```python
from build123d import *

# Parameters (mm, degrees)
SKETCH1_R           = 20
BOSS_EXTRUDE1_DEPTH = 30
SKETCH2_R           = 20
BOSS_EXTRUDE2_DEPTH = 5
SKETCH3_R           = 5.5
BOSS_EXTRUDE3_DEPTH = 5
FILLET1_R           = 10


with BuildPart() as part:
    # Sketch1 → Boss-Extrude1 (new body)
    with BuildSketch(Plane(origin=(0, 0, 0), x_dir=(1, 0, 0), z_dir=(0, 1, 0))):
        Circle(SKETCH1_R)
        with BuildLine():
            Line((-4.4, 17.6), (4.4, 17.6))
            Line((4.4, 17.6), (4.4, 12.073214154))
            ThreePointArc((4.4, 12.073214154), (0, -12.85), (-4.4, 12.073214154))
            Line((-4.4, 12.073214154), (-4.4, 17.6))
        make_face(mode=Mode.SUBTRACT)
    extrude(amount=BOSS_EXTRUDE1_DEPTH)

    # Sketch2 → Boss-Extrude2 (add)
    with BuildSketch(Plane(origin=(0, 30, 0), x_dir=(1, 0, 0), z_dir=(0, 1, 0))):
        Circle(SKETCH2_R)
    extrude(amount=BOSS_EXTRUDE2_DEPTH)

    # Sketch3 → Boss-Extrude3 (add)
    with BuildSketch(Plane(origin=(0, 35, 0), x_dir=(1, 0, 0), z_dir=(0, 1, 0))):
        Circle(SKETCH3_R)
        with BuildLine():
            Line((-2.71339271, 1.6), (2.71339271, 1.6))
            ThreePointArc((2.71339271, 1.6), (0, -3.15), (-2.71339271, 1.6))
        make_face(mode=Mode.SUBTRACT)
    extrude(amount=BOSS_EXTRUDE3_DEPTH)

    # Fillet1
    fillet1_edges = [part.edges().sort_by_distance(p)[0] for p in [
        (-20, 35, 0),
    ]]
    fillet(fillet1_edges, radius=FILLET1_R)


solid = part.part
```
Input: part model. Units: mm. Frame: model coordinates. A direction names the side the tool comes from. Give positions to 0.01 mm unless a question says otherwise; leave off trailing zeros. Write each loop counter-clockwise with the first axis right and the second up, starting at its lowest first coordinate (ties: lowest second). Pieces come first, ordered by that corner, then holes. Notation, with made-up numbers: (84, 70.5) - (98, 70.5) arc R28 ccw to (98, 106.5) - close; hole circle Ø3 at (31, 25). An arc over 180 degrees is marked (long way). Write item = value, one per line. Start each with the question number.
1. Ray query, L1, parallel to X at y = 14, z = 0; L2, parallel to Z at x = 0, y = 11.75; L3, parallel to Z at x = 0, y = 38.25. Return the intervals inside material, ascending.
2. First-contact query: pin 1 Ø15.5 at (x, z) = (0, 0) entering from -Y; pin 2 Ø5 at (x, z) = (10, -9.5) entering from +Y; pin 3 Ø4.5 at (x, y) = (1.5, 20.5) entering from +Z. Flat tips, straight axial feed; report the tip coordinate or a pass-through.
3. Access query for faces 5 (the cylindrical face through (0.09, 37.47, 3.15)), 6 (the flat face through (0, 15, -17.6)), 7 (the flat face through (-0.3, 0, 13.1)). Directions: +Z, -Z, +X, -X, +Y, -Y. A direction counts if a zero-diameter tool reaches every point of the face in a straight line with its end or side. Return the directions, or none.
4. Section query A-A, the plane y = 11. Output: boundary loops of the cut face in (x, z).
5. Mould query, pull axis X, two halves, no side actions, for faces 1 (the cylindrical face through (-4.336, 12.325, 19.524)), 2 (the cylindrical face through (0.5, 14.79, 12.84)), 3 (the flat face through (0, 30, -3)), 4 (the flat face through (0, 40, -3)). Classes: released by +X, released by -X, zero draft, split by the parting line, or undercut.
Check sheet entries:
q1.L1 = -20 to -12.85, 12.85 to 20
q1.L2 = -20 to -17.6, 12.85 to 20
q1.L3 = -5.5 to -1.6, 3.15 to 5.5
q2.pin_1 = 30
q2.pin_2 = 34.92
q2.pin_3 = 20
q3.face_5 = +Y
q3.face_6 = -Y
q3.face_7 = +Z, -Z, +X, -X, -Y
q4.outline = circle Ø40 at (0, 0); hole (-4.4, -17.6) - (4.4, -17.6) - (4.4, -12.07) arc R12.85 ccw (long way) to (-4.4, -12.07) - close
q5.face_1 = split by the parting line
q5.face_2 = undercut
q5.face_3 = undercut
q5.face_4 = zero draft
